from build123d import *

# Parameters (mm, degrees)
SKETCH1_W           = 170
SKETCH1_H           = 25
SKETCH1_R           = 2
SKETCH1_R_2         = 4.125
BOSS_EXTRUDE1_DEPTH = 4
SKETCH2_R           = 4.125
CUT_EXTRUDE1_DEPTH  = 87.007267135
SKETCH3_W           = 56.414472257
SKETCH3_H           = 25
SKETCH3_R           = 4.125
BOSS_EXTRUDE2_DEPTH = 9
FILLET1_R           = 40
SHELL2_T            = -3


with BuildPart() as part:
    # Sketch1 → Boss-Extrude1 (new body)
    with BuildSketch(Plane(origin=(0, 0, 0), x_dir=(1, 0, 0), z_dir=(0, 1, 0))):
        Rectangle(SKETCH1_W, SKETCH1_H)
        with Locations(Location((-28.158485727, -4.763382536, 0), (0, 0, 270))):
            Circle(SKETCH1_R, mode=Mode.SUBTRACT)
        with Locations(Location((6.841514273, -4.763382536, 0), (0, 0, 270))):
            Circle(SKETCH1_R, mode=Mode.SUBTRACT)
        with Locations(Location((72.5, 0, 0), (0, 0, 270))):
            Circle(SKETCH1_R_2, mode=Mode.SUBTRACT)
    extrude(amount=BOSS_EXTRUDE1_DEPTH)

    # Sketch2 → Cut-Extrude1 (cut, through all)
    with BuildSketch(Plane(origin=(0, 4, 0), x_dir=(1, 0, 0), z_dir=(0, 1, 0))):
        with Locations(Location((-72.5, 0, 0), (0, 0, 270))):
            Circle(SKETCH2_R)
    extrude(amount=-CUT_EXTRUDE1_DEPTH, mode=Mode.SUBTRACT)

    # Sketch3 → Boss-Extrude2 (add)
    with BuildSketch(Plane(origin=(0, 4, 0), x_dir=(1, 0, 0), z_dir=(0, 1, 0))):
        with Locations((56.792763872, 0)):
            Rectangle(SKETCH3_W, SKETCH3_H)
        with Locations(Location((72.5, 0, 0), (0, 0, 270))):
            Circle(SKETCH3_R, mode=Mode.SUBTRACT)
    extrude(amount=BOSS_EXTRUDE2_DEPTH)

    # Fillet1
    # the kernel refuses this fillet: 40 mm, written as the material it takes off along each edge
    with BuildSketch(Plane(origin=(28.585527743, 13, -75.696123299), x_dir=(1, 0, 0), z_dir=(0, 0, 1))) as fillet1_piece_1:
        with BuildLine():
            CenterArc((25.27844932, -40), FILLET1_R, 90, 39.194967426)
            Line((0, -9), (0, 0))
            Line((0, 0), (25.27844932, 0))
        make_face()
    extrude(amount=151.392246598, mode=Mode.SUBTRACT)

    # Shell2
    shell2_openings = [part.faces().sort_by_distance(p)[0] for p in [
        (85, 6.5, 0),
    ]]
    offset(amount=SHELL2_T, openings=shell2_openings)


solid = part.part
Model file for the job. Use its own axes, mm. A direction names the side the tool comes from. Give positions to 0.01 mm unless a question says otherwise; leave off trailing zeros. Loops run counter-clockwise (first coordinate to the right, second up) from the corner with the lowest first, then second, coordinate; pieces in that order, holes last. Notation, with made-up numbers: (18, 67) -> (71, 67) arc R14 cw to (71, 89) -> close; hole circle Ø7 at (80.5, 87). An arc over 180 degrees is marked (long way). Use a Markdown table: item, result. Add a question column.
(1) Tool access for faces 5 (the cylindrical face through (65.544, 6.451, -1.545)), 6 (the flat face through (64, 6, -9.5)), 7 (the cylindrical face through (8.824, 1.972, 4.503)): list every direction of +Z, -Z, +X, -X, +Y, -Y with a clear straight run to the whole face (end or side of a thin tool).
(2) Slice it at B-B on z = 0. List the corners of the cut face in (x, y) (3 decimals), and give its area (3 significant figures).
(3) Mould opens along Y. For faces 1 (the flat face through (-29, 4, 0)), 2 (the flat face through (66, 10, -4)), 3 (the flat face through (-85, 2, 0)), 4 (the flat face through (64, 6, 9.5)) say: +Y half, -Y half, draft (parallel to the pull), parting line (faces both ways), or undercut.
(4) Wall check: line 1 along X through (y, z) = (1.25, 0) (3 decimals); line 2 along Y through (x, z) = (66.5, 9); line 3 along X through (y, z) = (4.75, 1). Give the ranges that are in metal, low to high.
(5) Slice it at A-A on x = -72.5. List the corners of the cut face in (y, z) (3 decimals), and give its area (3 significant figures).
(6) Slice it at D-D on x = 35.5. List the corners of the cut face in (y, z).
(7) Drop flat-ended pins along their axis: pin 1 Ø6.5 at (x, z) = (72.5, 0) entering from -Y; pin 2 Ø4 at (x, z) = (37, -3.5) entering from +Y; pin 3 Ø1.5 at (x, z) = (22.5, -7) entering from -Y; pin 4 Ø9.5 at (x, z) = (45.5, 3.5) entering from +Y. Give the stop position or say it passes through.
(8) Slice it at C-C on x = 72.5. List the corners of the cut face in (y, z) (3 decimals), and give its area (4 significant figures).
Filled sheet:
| question | item | result |
|---|---|---|
| 1 | face 5 | none |
| 1 | face 6 | +X |
| 1 | face 7 | +Y, -Y |
| 2 | outline | (-85, 0) -> (-76.625, 0) -> (-76.625, 4) -> (-85, 4) -> close; (-68.375, 0) -> (68.375, 0) -> (68.375, 13) -> (53.864, 13) arc R40 ccw to (28.586, 4) -> (-68.375, 4) -> close; (76.625, 0) -> (85, 0) -> (85, 3) -> (79.625, 3) -> (79.625, 10) -> (85, 10) -> (85, 13) -> (76.625, 13) -> close; hole (32.208, 3) -> (65.375, 3) -> (65.375, 10) -> (53.864, 10) arc R37 ccw to start |
| 2 | area | 754 mm2 |
| 3 | face 1 | +Y half |
| 3 | face 2 | undercut |
| 3 | face 3 | draft |
| 3 | face 4 | undercut |
| 4 | line 1 | -85 to -76.625, -68.375 to 68.375, 76.625 to 85 |
| 4 | line 2 | 0 to 3, 10 to 13 |
| 4 | line 3 | 29.53 to 34.87, 65.45 to 68.5, 76.5 to 79.55 |
| 5 | outline | (0, -12.5) -> (4, -12.5) -> (4, -4.125) -> (0, -4.125) -> close; (0, 4.125) -> (4, 4.125) -> (4, 12.5) -> (0, 12.5) -> close |
| 5 | area | 67.0 mm2 |
| 6 | outline | (0, -12.5) -> (8.54, -12.5) -> (8.54, 12.5) -> (0, 12.5) -> close; hole (3, -9.5) -> (5.12, -9.5) -> (5.12, 9.5) -> (3, 9.5) -> close |
| 7 | pin 1 | through |
| 7 | pin 2 | y = 10.14 |
| 7 | pin 3 | y = 0 |
| 7 | pin 4 | y = 12.84 |
| 8 | outline | (0, -12.5) -> (13, -12.5) -> (13, -4.125) -> (0, -4.125) -> close; (0, 4.125) -> (13, 4.125) -> (13, 12.5) -> (0, 12.5) -> close; hole (3, -9.5) -> (10, -9.5) -> (10, -7.125) -> (3, -7.125) -> close; hole (3, 7.125) -> (10, 7.125) -> (10, 9.5) -> (3, 9.5) -> close |
| 8 | area | 184.5 mm2 |
